```python
from build123d import *

# Parameters (mm, degrees)
F1_DEPTH = 2.54
F2_SIZE  = 2.53999


# Not quite as in the source:
# - a fillet or chamfer is up to 0.001 mm smaller than in the source, because OpenCascade refuses the exact size


with BuildPart() as f1:
    # F0 (on Top) → F1 (new body)
    with BuildSketch(Plane.XY):
        with BuildLine():
            ThreePointArc((0, 25.4), (-9.009768429, 20.6793052869), (-19.05, 19.05))
            ThreePointArc((-19.05, 19.05), (-13.2442322719, -4.768956688), (0, -25.4))
            ThreePointArc((0, -25.4), (13.2442322719, -4.768956688), (19.05, 19.05))
            ThreePointArc((19.05, 19.05), (9.009768429, 20.6793052869), (0, 25.4))
        make_face()
    extrude(amount=F1_DEPTH)

    # F2 (size 2.54 in the source; OpenCascade refuses exactly that, so slightly less here)
    f2_edges = [f1.edges().sort_by_distance(p)[0] for p in [
        (13.244232, -4.768957, 0),
        (-13.244232, -4.768957, 0),
        (-9.009768, 20.679305, 0),
        (9.009768, 20.679305, 0),
    ]]
    chamfer(f2_edges, length=F2_SIZE)


solid = f1.part
```
CAD build for the part. Positions are in the model's coordinates, mm. Round coordinates to 2 decimals unless told otherwise and drop trailing zeros. Loops run counter-clockwise (first coordinate to the right, second up) from the corner with the lowest first, then second, coordinate; pieces in that order, holes last. Notation, with made-up numbers: (-27, 16.25) - (-22, 16.25) arc R15 ccw to (-22, 35.25) - close; hole circle Ø4 at (56.25, -23.75). An arc over 180 degrees is marked (long way). Return JSON: item names as keys, results as strings. Group by question number.
Q1. Flat gauge pin, fed straight in: pin 1 Ø1.5 at (x, z) = (-9, 2) entering from -Y. Where does the tip first touch, or does it go through?
Q2. Drill centre lines: line 1 along X through (y, z) = (13, 0.5); line 2 along Y through (x, z) = (-5.5, 0.6); line 3 along X through (y, z) = (-11.5, 1). Where is each one in solid material? Low to high. Write a range as [from, to].
Q3. Band-saw the part on A-A on z = 2.05. Give the cut face in (x, y), plus the area to 3 significant figures.
Solutions:
{
 "1": {"pin 1": "stops at y = -14.03"},
 "2": {"line 1": "x = [-16.29, 16.29]", "line 2": "y = [-15.12, 19.96]", "line 3": "x = [-8.18, 8.18]"},
 "3": {"outline": "(-18.52, 18.56) arc R73.78 ccw to (0, -24.67) arc R73.78 ccw to (18.52, 18.56) arc R32.24 cw to (0, 24.79) arc R32.24 cw to start", "area": "1,120 mm^2"}
}
